Design review of the part built by this model. Coordinates are the model's own, in mm. A direction names the side the tool comes from. Round coordinates to 2 decimals unless told otherwise and drop trailing zeros. Order: outer loops, then holes, each group sorted by start corner. A loop starts at its lowest first (then second) coordinate and runs counter-clockwise, first axis right, second up. Notation, with made-up numbers: M 65.25,19.25 L 96.25,19.25 A27 cw 96.25,52.25 Z; hole C -29,46.25 d1. An arc over 180 degrees is marked long. Write each question's results on one line, items separated by ' | '. Start each with the question number.
Item 1: Take a section at B-B, the plane z = 1.6. Write out the cut boundary in (x, y), plus the area to 3 significant figures.
Item 2: Wall thickness on line 1 (X direction, y = 16, z = 0.7); line 2 (X direction, y = 25.75, z = 2.55); line 3 (Y direction, x = 12.5, z = 2.2): over which ranges is each line inside the solid? List them lowest first. Write a range as [from, to].
Item 3: Clearance check with a flat-ended pin moving along its axis: pin 1 (6 mm diameter, centred on x = 6.5, y = 23.5, fed in from +Z). State where the tip first meets the part, or that it passes through.
Item 4: Take a section at C-C, the plane x = 7.5. Write out the cut boundary in (y, z), plus the area to 3 significant figures.
Item 5: Machinability: for faces 4 (the cylindrical face through (1.711, 28.196, 1.521)), 5 (the cylindrical face through (7.5, 2.5, 1.5)), which of the approach directions +Z, -Z, +X, -X, +Y, -Y give a long, thin tool a straight path to every point of the face, cutting with its end or side? Answer none if there is none.
Item 6: The part is to be moulded in two halves that separate along X. For faces 1 (the flat face through (9.5, 15, 1)), 2 (the flat face through (7, 30, 1)), 3 (the flat face through (15, 15, 1)), say which applies: +X half, -X half, draft (parallel to the pull), parting line (faces both ways), or undercut.
Item 7: Take a section at A-A, the plane y = 12.75. Write out the cut boundary in (x, z), plus the area to 3 significant figures.
Item 8: Take a section at D-D, the plane x = 13. Write out the cut boundary in (y, z), plus the area to 3 significant figures.
```python
from build123d import *

# Parameters (mm, degrees)
F0_W     = 15
F0_H     = 30
F1_DEPTH = 3
F2_R     = 6


with BuildPart() as f1:
    # F0 (on Top) → F1 (new body)
    with BuildSketch(Plane.XY):
        with Locations((7.5, 15)):
            Rectangle(F0_W, F0_H)
        with BuildLine():
            ThreePointArc((5.5, 25.5), (7.5, 27.5), (9.5, 25.5))
            Line((9.5, 25.5), (9.5, 4.5))
            ThreePointArc((9.5, 4.5), (7.5, 2.5), (5.5, 4.5))
            Line((5.5, 4.5), (5.5, 25.5))
        make_face(mode=Mode.SUBTRACT)
    extrude(amount=F1_DEPTH)

    # F2
    f2_edges = [f1.edges().sort_by_distance(p)[0] for p in [
        (15, 0, 1.5),
        (0, 0, 1.5),
        (15, 30, 1.5),
        (0, 30, 1.5),
    ]]
    fillet(f2_edges, radius=F2_R)


solid = f1.part
```
Results list:
1) outline: M 0,6 A6 ccw 6,0 L 9,0 A6 ccw 15,6 L 15,24 A6 ccw 9,30 L 6,30 A6 ccw 0,24 Z; hole M 5.5,4.5 A2 ccw 9.5,4.5 L 9.5,25.5 A2 ccw 5.5,25.5 Z | area: 323 mm²
2) line 1: [0, 5.5], [9.5, 15] | line 2: [0.26, 5.52], [9.48, 14.74] | line 3: [1.13, 28.87]
3) pin 1: z = 3
4) outline: M 0,0 L 2.5,0 L 2.5,3 L 0,3 Z; M 27.5,0 L 30,0 L 30,3 L 27.5,3 Z | area: 15.0 mm²
5) face 4: +Z, -Z, -X, +Y | face 5: +Z, -Z
6) face 1: undercut | face 2: draft | face 3: +X half
7) outline: M 0,0 L 5.5,0 L 5.5,3 L 0,3 Z; M 9.5,0 L 15,0 L 15,3 L 9.5,3 Z | area: 33.0 mm²
8) outline: M 1.53,0 L 28.47,0 L 28.47,3 L 1.53,3 Z | area: 80.8 mm²
